Build history of the part. All positions in model axes, mm. Face numbers are marked on the shaded views. A direction names the side the tool comes from. Coordinates: 2 decimals unless noted, no trailing zeros. Write each loop counter-clockwise with the first axis right and the second up, starting at its lowest first coordinate (ties: lowest second). Pieces come first, ordered by that corner, then holes. Notation, with made-up numbers: (71.25, 13) -> (124.25, 13) arc R29 ccw to (124.25, 40) -> close; hole circle Ø9 at (43.5, 67). An arc over 180 degrees is marked (long way). Write each question's results on one line, items separated by ' | '. Start each with the question number.
Q1. Tool access for the marked faces 4 and 5: list every direction of +Z, -Z, +X, -X, +Y, -Y with a clear straight run to the whole face (end or side of a thin tool).
Q2. Saw through at B-B on z = 6. Give the cut face in (x, y) (3 decimals).
Q3. Drop flat-ended pins along their axis: pin 1 Ø2.5 at (x, z) = (5.5, 6.5) entering from -Y; pin 2 Ø1 at (x, y) = (45.5, 4) entering from +Z; pin 3 Ø3.5 at (y, z) = (-13, 6) entering from -X. Give the stop position or say it passes through.
Q4. Two-plate mould, pull along Z, no slides. Class the marked faces 1, 2 and 3: released by +Z, released by -Z, zero draft, split by the parting line, or undercut.
Q5. Drill centre lines: line 1 (Z direction, x = 5, y = 0.25) (3 decimals); line 2 (Z direction, x = 4, y = -1.75); line 3 (Z direction, x = 12, y = 1.5). Where is each one in solid material? Low to high.
Q6. Saw through at C-C on y = -7. Give the cut face in (x, z) (3 decimals).
Q7. Saw through at A-A on x = 5. Give the cut face in (y, z) (3 decimals), and give its area (3 significant figures).
Q8. Saw through at D-D on x = 29.25. Give the cut face in (y, z), and give its area (3 significant figures).
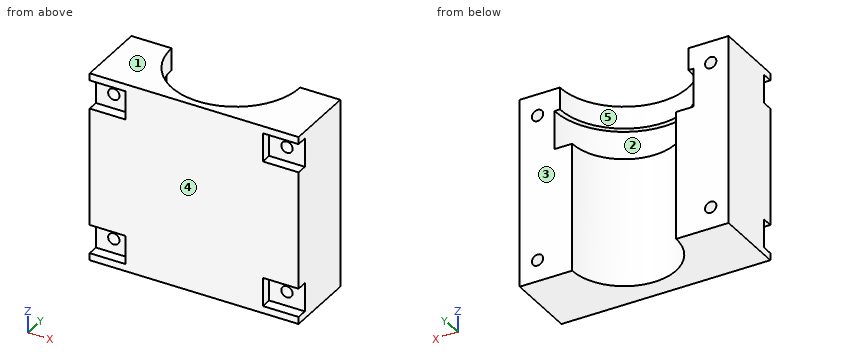
from build123d import *

# Parameters (mm, degrees)
SKETCH1_W                                  = 58.5
SKETCH1_H                                  = 20
BOSS_EXTRUDE1_DEPTH                        = 53
CUT_EXTRUDE2_DEPTH                         = 17
CUT_EXTRUDE3_DEPTH                         = 42.5
SKETCH8_W                                  = 10
SKETCH8_H                                  = 8
CUT_EXTRUDE6_DEPTH                         = 3
SKETCH7_R                                  = 1.585
CUT_EXTRUDE5_DEPTH                         = 92.5
MIRROR1_AT_THE_SECOND_PLANE_COPY_1_SKETC_W = 10
MIRROR1_AT_THE_SECOND_PLANE_COPY_1_SKETC_H = 8
MIRROR1_AT_THE_SECOND_PLANE_COPY_1_DEPTH   = 3
CUT_EXTRUDE7_DEPTH                         = 10.8


with BuildPart() as part:
    # Sketch1 → Boss-Extrude1 (new body)
    with BuildSketch(Plane.XY):
        with Locations((29.25, -3.609195402)):
            Rectangle(SKETCH1_W, SKETCH1_H)
    extrude(amount=BOSS_EXTRUDE1_DEPTH)

    # Sketch3 → Cut-Extrude2 (cut)
    with BuildSketch(Plane.XY.offset(53)):
        with BuildLine():
            Line((11.25, 6.390804598), (47.25, 6.390804598))
            ThreePointArc((47.25, 6.390804598), (29.25, -11.609195402), (11.25, 6.390804598))
        make_face()
    extrude(amount=-CUT_EXTRUDE2_DEPTH, mode=Mode.SUBTRACT)

    # Sketch5 → Cut-Extrude3 (cut)
    with BuildSketch(Plane(origin=(0, 0, 0), x_dir=(-1, 0, 0), z_dir=(0, 0, -1))):
        with BuildLine():
            Line((-43.8, 6.390804598), (-14.7, 6.390804598))
            ThreePointArc((-14.7, 6.390804598), (-29.25, -8.159195402), (-43.8, 6.390804598))
        make_face()
    extrude(amount=-CUT_EXTRUDE3_DEPTH, mode=Mode.SUBTRACT)

    # Sketch8 → Cut-Extrude6 (cut)
    with BuildSketch(Plane(origin=(0, -13.609195402, 0), x_dir=(-1, 0, 0), z_dir=(0, -1, 0))):
        with Locations((-53.5, -6)):
            Rectangle(SKETCH8_W, SKETCH8_H)
    cut_extrude6 = extrude(amount=-CUT_EXTRUDE6_DEPTH, mode=Mode.SUBTRACT)

    # Sketch7 → Cut-Extrude5 (cut)
    with BuildSketch(Plane(origin=(0, -13.609195402, 0), x_dir=(-1, 0, 0), z_dir=(0, -1, 0))):
        with Locations(Location((-53.5, -47, 0), (0, 0, 180))):
            Circle(SKETCH7_R)
        with Locations(Location((-53.5, -6, 0), (0, 0, 180))):
            Circle(SKETCH7_R)
        with Locations(Location((-5, -6, 0), (0, 0, 180))):
            Circle(SKETCH7_R)
        with Locations(Location((-5, -47, 0), (0, 0, 180))):
            Circle(SKETCH7_R)
    extrude(amount=-CUT_EXTRUDE5_DEPTH, mode=Mode.SUBTRACT)

    # Mirror1: Cut-Extrude6 across plane
    add(cut_extrude6.mirror(Plane.XY.offset(26.5)), mode=Mode.SUBTRACT)

    # Mirror1 at the second plane: Cut-Extrude6 across plane
    add(cut_extrude6.mirror(Plane.ZY.offset(-29.25)), mode=Mode.SUBTRACT)

    # Mirror1 at the second plane copy 1 sketc → Mirror1 at the second plane copy 1 (cut)
    with BuildSketch(Plane(origin=(58.5, -13.609195402, 53), x_dir=(1, 0, 0), z_dir=(0, -1, 0))):
        with Locations((-53.5, -6)):
            Rectangle(MIRROR1_AT_THE_SECOND_PLANE_COPY_1_SKETC_W, MIRROR1_AT_THE_SECOND_PLANE_COPY_1_SKETC_H)
    extrude(amount=-MIRROR1_AT_THE_SECOND_PLANE_COPY_1_DEPTH, mode=Mode.SUBTRACT)

    # Sketch11 → Cut-Extrude7 (cut)
    with BuildSketch(Plane.XY.offset(36)):
        with BuildLine():
            Line((9.75, 6.390804598), (48.75, 6.390804598))
            ThreePointArc((48.75, 6.390804598), (29.25, -13.109195402), (9.75, 6.390804598))
        make_face()
    extrude(amount=CUT_EXTRUDE7_DEPTH, mode=Mode.SUBTRACT)


solid = part.part
Returned:
1) face 4: +Z, -Z, +X, -X, -Y | face 5: +Z, +Y
2) outline: (0, -10.609) -> (3.415, -10.609) -> (3.415, 6.391) -> (0, 6.391) -> close; (6.585, -10.609) -> (10, -10.609) -> (10, -13.609) -> (48.5, -13.609) -> (48.5, -10.609) -> (51.915, -10.609) -> (51.915, 6.391) -> (43.8, 6.391) arc R14.55 cw to (14.7, 6.391) -> (6.585, 6.391) -> close; (55.085, -10.609) -> (58.5, -10.609) -> (58.5, 6.391) -> (55.085, 6.391) -> close
3) pin 1: stops at y = -10.61 | pin 2: stops at z = 36 | pin 3: stops at x = 10
4) face 1: released by +Z | face 2: undercut | face 3: zero draft
5) line 1: z = 0 to 4.415, 7.585 to 45.415, 48.585 to 53 | line 2: z = 0 to 4.77, 7.23 to 45.77, 48.23 to 53 | line 3: z = 0 to 36
6) outline: (0, 0) -> (23.559, 0) -> (23.559, 36) -> (15.075, 36) -> (15.075, 46.8) -> (17.221, 46.8) -> (17.221, 53) -> (0, 53) -> close; (34.941, 0) -> (58.5, 0) -> (58.5, 53) -> (41.279, 53) -> (41.279, 46.8) -> (43.425, 46.8) -> (43.425, 36) -> (34.941, 36) -> close; hole circle Ø3.17 at (5, 6); hole circle Ø3.17 at (5, 47); hole circle Ø3.17 at (53.5, 6); hole circle Ø3.17 at (53.5, 47)
7) outline: (-13.609, 0) -> (6.391, 0) -> (6.391, 4.415) -> (-10.609, 4.415) -> (-10.609, 2) -> (-13.609, 2) -> close; (-13.609, 10) -> (-10.609, 10) -> (-10.609, 7.585) -> (6.391, 7.585) -> (6.391, 45.415) -> (-10.609, 45.415) -> (-10.609, 43) -> (-13.609, 43) -> close; (-13.609, 51) -> (-10.609, 51) -> (-10.609, 48.585) -> (6.391, 48.585) -> (6.391, 53) -> (-13.609, 53) -> close | area: 904 mm2
8) outline: (-13.61, 0) -> (-8.16, 0) -> (-8.16, 36) -> (-13.11, 36) -> (-13.11, 46.8) -> (-11.61, 46.8) -> (-11.61, 53) -> (-13.61, 53) -> close | area: 214 mm2
